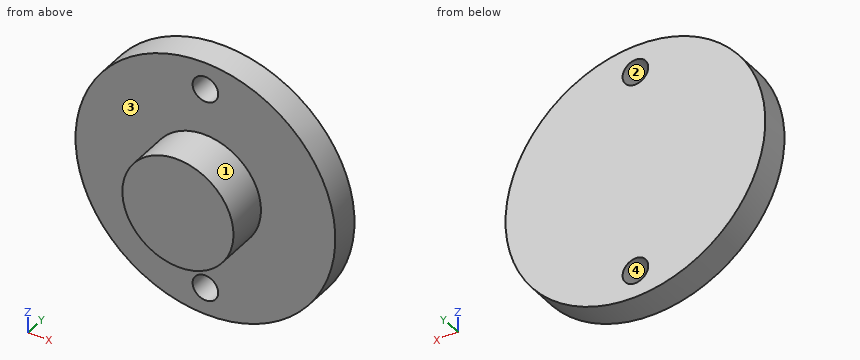
```python
from build123d import *

# Parameters (mm, degrees)
SKETCH1_R           = 10.287
BOSS_EXTRUDE1_DEPTH = 2.3
SKETCH2_R           = 4.4
BOSS_EXTRUDE2_DEPTH = 3.3
SKETCH4_R           = 1.016
CUT_EXTRUDE1_DEPTH  = 2.3


with BuildPart() as part:
    # Sketch1 → Boss-Extrude1 (new body)
    with BuildSketch(Plane(origin=(0, 0, 0), x_dir=(1, 0, 0), z_dir=(0, 1, 0))):
        with Locations(Location((0, 0, 0), (0, 0, 270))):
            Circle(SKETCH1_R)
    extrude(amount=BOSS_EXTRUDE1_DEPTH)

    # Sketch2 → Boss-Extrude2 (add)
    with BuildSketch(Plane(origin=(0, 0, 0), x_dir=(-1, 0, 0), z_dir=(0, -1, 0))):
        with Locations(Location((0, 0, 0), (0, 0, 90))):
            Circle(SKETCH2_R)
    extrude(amount=BOSS_EXTRUDE2_DEPTH)

    # Sketch4 → Cut-Extrude1 (cut)
    with BuildSketch(Plane(origin=(0, 0, 0), x_dir=(1, 0, 0), z_dir=(0, 1, 0))):
        with Locations(Location((0, 8.128, 0), (0, 0, 270))):
            Circle(SKETCH4_R)
        with Locations(Location((0, -8.128, 0), (0, 0, 270))):
            Circle(SKETCH4_R)
    extrude(amount=CUT_EXTRUDE1_DEPTH, mode=Mode.SUBTRACT)


solid = part.part
```
The model under review builds one solid part; all positions refer to its coordinate system, in mm. Face numbers are marked on the shaded views. Coordinates: 2 decimals unless noted, no trailing zeros. Write each loop counter-clockwise with the first axis right and the second up, starting at its lowest first coordinate (ties: lowest second). Pieces come first, ordered by that corner, then holes.
1) We need section A-A on x = 0. State the section outline as (y, z) points.
2) We need section C-C on y = 0.6. State the section outline as (x, z) points, then the cut area to 3 significant figures.
3) The part is to be moulded in two halves that separate along X. For the marked faces 1, 2, 3 and 4, say which applies: pulls with the +X half, pulls with the -X half, needs draft (parallel to the pull), parting line crosses it, or undercut.
4) We need section B-B on z = 0. State the section outline as (x, y) points.
5) We need section D-D on z = -8. State the section outline as (x, y) points.
6) To check wall thickness, follow probe 1 along Y at (x, z) = (-2, -9); probe 2 along X at (y, z) = (0.05, -9); probe 3 along Z at (x, y) = (-2.5, 0.45). State the ranges of each line that lie inside material, in increasing order.
7) Clearance check with flat-ended pins moving along their axes: pin 1 Ø1 at (x, z) = (1.5, 6) entering from -Y; pin 2 Ø1 at (x, y) = (3, 1) entering from -Z; pin 3 Ø3 at (x, y) = (-7.5, -0.5) entering from -Z. State where each tip first meets the part, or that it passes through.
Answer list:
1. outline: (-3.3, -4.4) - (0, -4.4) - (0, -7.11) - (2.3, -7.11) - (2.3, 7.11) - (0, 7.11) - (0, 4.4) - (-3.3, 4.4) - close; (0, -10.29) - (2.3, -10.29) - (2.3, -9.14) - (0, -9.14) - close; (0, 9.14) - (2.3, 9.14) - (2.3, 10.29) - (0, 10.29) - close
2. outline: circle Ø20.57 at (0, 0); hole circle Ø2.03 at (0, -8.13); hole circle Ø2.03 at (0, 8.13)
2. area: 326 mm2
3. face 1: parting line crosses it
3. face 2: undercut
3. face 3: needs draft
3. face 4: undercut
4. outline: (-10.29, 0) - (-4.4, 0) - (-4.4, -3.3) - (4.4, -3.3) - (4.4, 0) - (10.29, 0) - (10.29, 2.3) - (-10.29, 2.3) - close
5. outline: (-6.47, 0) - (-1.01, 0) - (-1.01, 2.3) - (-6.47, 2.3) - close; (1.01, 0) - (6.47, 0) - (6.47, 2.3) - (1.01, 2.3) - close
6. probe 1: y = 0 to 2.3
6. probe 2: x = -4.98 to -0.52, 0.52 to 4.98
6. probe 3: z = -9.98 to 9.98
7. pin 1: stops at y = 0
7. pin 2: stops at z = -9.98
7. pin 3: stops at z = -8.29
